Autodesk Inventor part; units mm, degrees
ref_plane "Work Plane1" through (-26.7016, -22.7609, 2.3) normal (0, 0, 1) x (1, 0, 0)
ref_plane "YZ Plane" through (0, 0, 0) normal (1, 0, 0) x (0, 1, 0)
ref_plane "XZ Plane" through (0, 0, 0) normal (0, 1, 0) x (-1, 0, 0)
sketch "Sketch1" plane through (0, 0, 0) normal (0, 0, 1) x (1, 0, 0)
  line L0 (17.4, 4.3375) -> (19.4, 4.3375)
  line L1 (19.4, 8.4) -> (19.4, 4.3375)
  arc A0 (19.4, 8.4) -> (18.4, 9.4) centre (18.4, 8.4) ccw
  line L2 (-18.4, 9.4) -> (18.4, 9.4)
  arc A1 (-18.4, 9.4) -> (-19.4, 8.4) centre (-18.4, 8.4) ccw
  line L3 (-19.4, -8.4) -> (-19.4, 8.4)
  arc A2 (-19.4, -8.4) -> (-18.4, -9.4) centre (-18.4, -8.4) ccw
  line L4 (18.4, -9.4) -> (-18.4, -9.4)
  arc A3 (18.4, -9.4) -> (19.4, -8.4) centre (18.4, -8.4) ccw
  line L5 (19.4, -4.2375) -> (19.4, -8.4)
  line L6 (19.4, -4.2375) -> (17.4, -4.2375)
  arc A4 (17.4, -4.2375) -> (14.1485, -7.6) centre (20.15, -10.15) ccw
  line L7 (14.1485, -7.6) -> (-14.247, -7.6)
  arc A5 (-14.247, -7.6) -> (-17.4, -4.3375) centre (-20.15, -10.15) ccw
  line L8 (-17.4, -4.3375) -> (-17.4, 4.2375)
  arc A6 (-17.4, 4.2375) -> (-14.1485, 7.6) centre (-20.15, 10.15) ccw
  line L9 (-14.1485, 7.6) -> (14.247, 7.6)
  arc A7 (14.247, 7.6) -> (17.4, 4.3375) centre (20.15, 10.15) ccw
  circle A8 centre (-17.9, -7.9) radius 1
  circle A9 centre (17.9, -7.9) radius 1
  circle A10 centre (-17.9, 7.9) radius 1
  circle A11 centre (17.9, 7.9) radius 1
  line L10 (19.4, -2.5) -> (19.4, 2.5)
  line L11 (19.4, 8.4) -> (19.4, 2.5)
  line L12 (19.4, -2.5) -> (19.4, -8.4)
  point P0 (0, 0)
ref_plane "Work Plane1" through (-26.7016, -22.7609, 2.3) normal (0, 0, 1) x (1, 0, 0)
extrude "Extrusion1" add sketch "Sketch1" along normal up to surface (2.3 mm away) contours A7 L9 A6 L8 A5 L7 A4 L6 L5 A3 L4 A2 L3 A1 L2 A0 L1 L0
sketch "Sketch2" plane through (0, 0, 0) normal (0, 0, -1) x (-1, 0, 0)
  arc A0 (14.1485, 7.6) -> (17.4, 4.2375) centre (20.15, 10.15) ccw
  line L0 (17.4, -4.3375) -> (17.4, 4.2375)
  arc A1 (17.4, -4.3375) -> (14.247, -7.6) centre (20.15, -10.15) ccw
  line L1 (-14.1485, -7.6) -> (14.247, -7.6)
  arc A2 (-14.1485, -7.6) -> (-17.4, -4.2375) centre (-20.15, -10.15) ccw
  line L2 (-17.4, -4.2375) -> (-19.4, -4.2375)
  line L3 (-19.4, -4.2375) -> (-19.4, 4.3375)
  line L4 (-19.4, 4.3375) -> (-17.4, 4.3375)
  arc A3 (-17.4, 4.3375) -> (-14.247, 7.6) centre (-20.15, 10.15) ccw
  line L5 (14.1485, 7.6) -> (-14.247, 7.6)
  point P0 (0, 0)
extrude "Extrusion2" add sketch "Sketch2" along normal blind 1.5
sketch "Sketch3" plane through (0, 0, 0) normal (0, 0, 1) x (1, 0, 0)
  line L0 (19.4, 4.3375) -> (19.4, -4.2375)
  line L1 (17.4, 4.3375) -> (19.4, 4.3375)
  arc A0 (14.247, 7.6) -> (17.4, 4.3375) centre (20.15, 10.15) ccw
  line L2 (-14.1485, 7.6) -> (14.247, 7.6)
  arc A1 (-17.4, 4.2375) -> (-14.1485, 7.6) centre (-20.15, 10.15) ccw
  line L3 (-17.4, -4.3375) -> (-17.4, 4.2375)
  arc A2 (-14.247, -7.6) -> (-17.4, -4.3375) centre (-20.15, -10.15) ccw
  line L4 (14.1485, -7.6) -> (-14.247, -7.6)
  arc A3 (17.4, -4.2375) -> (14.1485, -7.6) centre (20.15, -10.15) ccw
  line L5 (19.4, -4.2375) -> (17.4, -4.2375)
  arc A4 (13.332, 6.1) -> (17.0815, 2.8375) centre (20.15, 10.15) ccw
  line L6 (17.0815, 2.8375) -> (17.9, 2.8375)
  line L7 (17.9, 2.8375) -> (17.9, -2.7375)
  line L8 (17.9, -2.7375) -> (17.0861, -2.7375)
  arc A5 (17.0861, -2.7375) -> (13.2269, -6.1) centre (20.15, -10.15) ccw
  line L9 (13.2269, -6.1) -> (-13.332, -6.1)
  arc A6 (-13.332, -6.1) -> (-15.9, -3.4548) centre (-20.15, -10.15) ccw
  line L10 (-15.9, -3.4548) -> (-15.9, 3.3478)
  arc A7 (-15.9, 3.3478) -> (-13.2269, 6.1) centre (-20.15, 10.15) ccw
  line L11 (-13.2269, 6.1) -> (13.332, 6.1)
  line L12 (17.9, 2.8375) -> (19.4, 2.8375)
  line L13 (19.4, 2.8375) -> (19.4, -2.7375)
  line L14 (19.4, -2.7375) -> (17.9, -2.7375)
  line L15 (17.9, -2.7375) -> (17.9, 2.8375)
  point P0 (0, 0)
  dimension "d4" = 1.5
  dimension "d5" = 5.575
extrude "Extrusion3" add sketch "Sketch3" along normal up to surface (2.3 mm away) contours L0 L12 L6 A4 L11 A7 L10 A6 L9 A5 L8 L14 L5 A3 L4 A2 L3 A1 L2 A0 L1
sketch "Sketch4" plane through (-18.4, 9.4, 2.3) normal (0, 0, 1) x (1, 0, 0)
  line L0 (37.8, -12.1375) -> (37.8, -17.8)
  line L1 (35.4861, -12.1375) -> (37.8, -12.1375)
  arc A0 (35.4861, -12.1375) -> (31.6269, -15.5) centre (38.55, -19.55) ccw
  line L2 (5.068, -15.5) -> (31.6269, -15.5)
  arc A1 (5.068, -15.5) -> (2.5, -12.8548) centre (-1.75, -19.55) ccw
  line L3 (2.5, -6.0522) -> (2.5, -12.8548)
  arc A2 (2.5, -6.0522) -> (5.1731, -3.3) centre (-1.75, 0.75) ccw
  line L4 (31.732, -3.3) -> (5.1731, -3.3)
  arc A3 (31.732, -3.3) -> (35.4815, -6.5625) centre (38.55, 0.75) ccw
  line L5 (37.8, -6.5625) -> (35.4815, -6.5625)
  line L6 (37.8, -1) -> (37.8, -6.5625)
  arc A4 (37.8, -1) -> (36.8, 0) centre (36.8, -1) ccw
  line L7 (0, 0) -> (36.8, 0)
  arc A5 (0, 0) -> (-1, -1) centre (0, -1) ccw
  line L8 (-1, -17.8) -> (-1, -1)
  arc A6 (-1, -17.8) -> (0, -18.8) centre (0, -17.8) ccw
  line L9 (36.8, -18.8) -> (0, -18.8)
  arc A7 (36.8, -18.8) -> (37.8, -17.8) centre (36.8, -17.8) ccw
  arc A8 (37.45, -1) -> (36.8, -0.35) centre (36.8, -1) ccw
  line L10 (37.45, -1) -> (37.45, -6.2125)
  line L11 (37.45, -6.2125) -> (35.5528, -6.2125)
  arc A9 (31.9342, -2.95) -> (35.5528, -6.2125) centre (38.55, 0.75) ccw
  line L12 (31.9342, -2.95) -> (4.9694, -2.95)
  arc A10 (2.15, -5.8553) -> (4.9694, -2.95) centre (-1.75, 0.75) ccw
  line L13 (2.15, -5.8553) -> (2.15, -13.05)
  arc A11 (4.8658, -15.85) -> (2.15, -13.05) centre (-1.75, -19.55) ccw
  line L14 (4.8658, -15.85) -> (31.8306, -15.85)
  arc A12 (35.5564, -12.4875) -> (31.8306, -15.85) centre (38.55, -19.55) ccw
  line L15 (35.5564, -12.4875) -> (37.45, -12.4875)
  line L16 (37.45, -12.4875) -> (37.45, -17.8)
  arc A13 (36.8, -18.45) -> (37.45, -17.8) centre (36.8, -17.8) ccw
  line L17 (36.8, -18.45) -> (0, -18.45)
  arc A14 (-0.65, -17.8) -> (0, -18.45) centre (0, -17.8) ccw
  line L18 (-0.65, -17.8) -> (-0.65, -1)
  arc A15 (0, -0.35) -> (-0.65, -1) centre (0, -1) ccw
  line L19 (0, -0.35) -> (36.8, -0.35)
  line L20 (37.45, -6.2125) -> (37.45, -12.4875)
  line L21 (37.8, -6.5625) -> (37.8, -12.1375)
  line L22 (37.8, -6.2125) -> (37.8, -1)
  arc A16 (37.8, -1) -> (36.8, 0) centre (36.8, -1) ccw
  line L23 (36.8, 0) -> (0, 0)
  arc A17 (0, 0) -> (-1, -1) centre (0, -1) ccw
  line L24 (-1, -1) -> (-1, -17.8)
  arc A18 (-1, -17.8) -> (0, -18.8) centre (0, -17.8) ccw
  line L25 (0, -18.8) -> (36.8, -18.8)
  arc A19 (36.8, -18.8) -> (37.8, -17.8) centre (36.8, -17.8) ccw
  line L26 (37.8, -17.8) -> (37.8, -12.4875)
  line L27 (37.8, -6.2125) -> (37.8, -12.4875)
  line L28 (-1, 0) -> (37.8, 0)
  line L29 (37.8, 0) -> (37.8, -18.8)
  line L30 (37.8, -18.8) -> (-1, -18.8)
  line L31 (-1, -18.8) -> (-1, 0)
  line L32 (-0.65, -0.35) -> (37.45, -0.35)
  line L33 (37.45, -0.35) -> (37.45, -18.45)
  line L34 (37.45, -18.45) -> (-0.65, -18.45)
  line L35 (-0.65, -18.45) -> (-0.65, -0.35)
  point P0 (18.4, -9.4)
  dimension "d8" = 0.35
  dimension "d9" = 0
extrude "Extrusion4" cut sketch "Sketch4" against normal up to surface (2.3 mm away) contours L0 A7 L9 A6 L8 A5 L7 A4 L6 L5 L20 L10 L33 L32 L19 L35 L18 L34 L17 L16 L1 | L20 L15 A12 L14 A11 L13 A10 L12 A9 L11 L5 A3 L4 A2 L3 A1 L2 A0 L1 | L33 L34 A13 | A8 L32 L33 | L34 L35 A14 | A15 L35 L32
properties part number "contramoldetapasevo"
Input: part model. Units: mm. Frame: model coordinates. A direction names the side the tool comes from. Give positions to 0.01 mm unless a question says otherwise; leave off trailing zeros. Write each loop counter-clockwise with the first axis right and the second up, starting at its lowest first coordinate (ties: lowest second). Pieces come first, ordered by that corner, then holes. Notation, with made-up numbers: M 15,6.25 L 64,6.25 A29 ccw 64,37.25 Z; hole C 10.25,79.5 d11. An arc over 180 degrees is marked long. Use one line per item in the form item = value.
1. Cut plane C-C on z = -0.65. Return loops of the section in (x, y), and give its area (3 significant figures).
Outcome:
outline = M -17.4,-4.34 A6.43 cw -14.25,-7.6 L 14.15,-7.6 A6.52 cw 17.4,-4.24 L 19.4,-4.24 L 19.4,4.34 L 17.4,4.34 A6.43 cw 14.25,7.6 L -14.15,7.6 A6.52 cw -17.4,4.24 Z
area = 520 mm²
2. Reachability of faces 4 (the face through (0, -7.6, -1)), 5 (the face through (-2, 8, 0)), 6 (the face through (0, -6.45, 1)) from +Z, -Z, +X, -X, +Y, -Y: full face, straight path, thin tool, end or side. Return the list, or none.
Outcome:
face_4 = -Z, +X, -X, -Y
face_5 = -Z
face_6 = +Z
3. Cut plane D-D on y = 0. Return loops of the section in (x, z), and give its area (3 significant figures).
Outcome:
outline = M -19.05,0 L -17.4,0 L -17.4,-1.5 L 19.4,-1.5 L 19.4,0 L -16.25,0 L -16.25,2.3 L -19.05,2.3 Z
area = 61.6 mm²
4. Cut plane B-B on z = 1.2. Return loops of the section in (x, y).
Outcome:
outline = M -19.05,-8.4 A0.65 ccw -18.4,-9.05 L 18.4,-9.05 A0.65 ccw 19.05,-8.4 L 19.05,-3.09 L 17.16,-3.09 A7.67 ccw 13.43,-6.45 L -13.53,-6.45 A7.58 ccw -16.25,-3.65 L -16.25,3.54 A7.67 ccw -13.43,6.45 L 13.53,6.45 A7.58 ccw 17.15,3.19 L 19.05,3.19 L 19.05,8.4 A0.65 ccw 18.4,9.05 L -18.4,9.05 A0.65 ccw -19.05,8.4 Z; hole C -17.9,-7.9 d2; hole C -17.9,7.9 d2; hole C 17.9,-7.9 d2; hole C 17.9,7.9 d2
5. Mould query, pull axis X, two halves, no side actions, for faces 1 (the face through (19.05, 6, 1)), 2 (the face through (-16.976, -7.517, 1.134)), 3 (the face through (18, -4.238, -1)). Classes: released by +X, released by -X, zero draft, split by the parting line, or undercut.
Outcome:
face_1 = released by +X
face_2 = undercut
face_3 = zero draft
6. Cut plane A-A on x = 17.9. Return loops of the section in (y, z).
Outcome:
outline = M -9.05,0 L -8.9,0 L -8.9,2.3 L -9.05,2.3 Z; M -6.9,0 L -4.24,0 L -4.24,-1.5 L 4.34,-1.5 L 4.34,0 L 6.9,0 L 6.9,2.3 L 3.19,2.3 L 3.19,0 L -3.09,0 L -3.09,2.3 L -6.9,2.3 Z; M 8.9,0 L 9.05,0 L 9.05,2.3 L 8.9,2.3 Z
7. First-contact query: P1, Ø2.5, axis at x = -17.9, y = -7.9, coming from the +Z side; P2, Ø3, axis at x = 17.9, y = 7.9, coming from the -Z side; P3, Ø1.8, axis at y = -7, z = 1.5, coming from the +X side; P4, Ø6.5, axis at x = 1.5, y = 1, coming from the +Z side. Flat tips, straight axial feed; report the tip coordinate or a pass-through.
Outcome:
P1 = 2.3
P2 = 0
P3 = 19.05
P4 = 0
8. Ray query, L1, parallel to Y at x = 17.9, z = 0.6; L2, parallel to Y at x = -17.9, z = 0.55; L3, parallel to Y at x = 0, z = 2.1. Return the intervals inside material, ascending.
Outcome:
L1 = -9.05 to -8.9, -6.9 to -3.09, 3.19 to 6.9, 8.9 to 9.05
L2 = -9.05 to -8.9, -6.9 to 6.9, 8.9 to 9.05
L3 = -9.05 to -6.45, 6.45 to 9.05
